Autodesk Inventor part; units mm, degrees
ref_plane "YZ Plane" through (0, 0, 0) normal (1, 0, 0) x (0, 1, 0)
ref_plane "XZ Plane" through (0, 0, 0) normal (0, 1, 0) x (-1, 0, 0)
ref_plane "XY Plane" through (0, 0, 0) normal (0, 0, 1) x (1, 0, 0)
sketch "スケッチ1" plane through (0, 0, 0) normal (0, 0, 1) x (1, 0, 0)
  line L0 (-28, -21) -> (28.6, -21)
  line L1 (28.6, -21) -> (28.6, 21)
  line L2 (28.6, 21) -> (-28, 21)
  line L3 (-28, 21) -> (-28, -21)
  point P0 (0, 0)
  dimension "d1" = 42
  dimension "d28" = 28
  dimension "d29" = 28.6
  dimension "d32" = 21
extrude "プレート1" add sketch "スケッチ1" along normal blind 2
sketch "スケッチ2" plane through (0, 0, 2) normal (0, 0, 1) x (1, 0, 0)
  line L0 (-24, -5) -> (24.6, -5)
  line L1 (24.6, -5) -> (24.6, 5)
  line L2 (24.6, 5) -> (-24, 5)
  line L3 (-24, 5) -> (-24, -5)
  line L4 (-24, -5) -> (24.6, 5) construction
  line L5 (24.6, -5) -> (-24, 5) construction
  line L6 (28.6, -21) -> (-28, -21)
  line L7 (-28, -21) -> (-28, 21)
  line L8 (28.6, -21) -> (-28, -21)
  line L9 (28.6, 21) -> (28.6, -21)
  line L10 (-28, 21) -> (28.6, 21)
  circle A0 centre (-10, 0) radius 7
  point P0 (0.3, 0)
  point P1 (0.3, 0)
  point P2 (0.3, 0)
  point P3 (0, 0)
  dimension "d3" = 48.6
  dimension "d5" = 10
  dimension "d16" = 14
  dimension "d31" = 14
  dimension "d33" = 4
  dimension "d34" = 0
hole "穴1" at (24.6, 5, 2) at (24.6, -5, 2) at (-24, 5, 2) at (-24, -5, 2) direction (0, 0, -1) diameter 4.3 end through all
extrude "押し出し1" cut sketch "スケッチ2" against normal blind 10 contours A0 L2 L0 | L0 A0 | A0 L2
sketch "スケッチ3" plane through (0, 0, 2) normal (0, 0, 1) x (1, 0, 0)
  line L0 (-28, 21) -> (28.6, 21)
  line L1 (-28, -21) -> (-28, 21)
  line L2 (28.6, -21) -> (-28, -21)
  line L3 (28.6, 21) -> (28.6, -21)
  line L4 (24.6, 17) -> (-24, 17)
  line L5 (-24, 17) -> (-24, -17)
  line L6 (-24, -17) -> (24.6, -17)
  line L7 (24.6, -17) -> (24.6, 17)
  point P0 (0, 0)
  dimension "d19" = 4
hole "穴2" at (-24, 17, 2) at (-24, -17, 2) at (24.6, 17, 2) at (24.6, -17, 2) direction (0, 0, -1) diameter 4.3 end through all
fillet "コーナーR1" radius 4 4 edges at (28.6, 21, 1) (-28, 21, 1) (-28, -21, 1) (28.6, -21, 1)
equation "\"d14\" = Thickness"
equation "\"d2\" = Thickness"
equation "\"BendRadius\" = Thickness"
equation "\"BendReliefWidth\" = Thickness"
equation "\"BendReliefDepth\" = 0.5 * Thickness"
equation "\"CornerReliefSize\" = 4 * Thickness"
equation "\"MinimumRemnant\" = 2 * Thickness"
equation "\"TransitionRadius\" = BendRadius"
equation "\"JacobiRadiusSize\" = BendRadius"
equation "\"GapSize\" = Thickness"
properties part number "s_carbon_plate4" material "CFRP"
Could you check a few things on this model? Use its own coordinates, in mm. Coordinates: 2 decimals unless noted, no trailing zeros. Loops run counter-clockwise (first coordinate to the right, second up) from the corner with the lowest first, then second, coordinate; pieces in that order, holes last. Notation, with made-up numbers: M -15.75,67 L 22.25,67 A16 ccw 22.25,95 Z; hole C 58.25,-9.5 d7. An arc over 180 degrees is marked long. Put each result on its own line as item: value. Start each with the question number.
(1) Thinking about a two-plate mould opening in X: for faces 1 (the face through (27.397, -19.859, 1.014)), 2 (the face through (0, 0, 2)), 3 (the face through (-3.534, -2.681, 1.014)), which applies, pulls with the +X half, pulls with the -X half, needs draft (parallel to the pull), parting line crosses it, or undercut?
(2) I need wall thicknesses on line 1 (X direction, y = -17, z = 1.4); line 2 (Y direction, x = -24, z = 1.1); line 3 (X direction, y = -5, z = 0.55). Which ranges of each line are inside material? Lowest first, please. Write a range as from..to.
(3) Suppose I cut it at C-C on y = -5. Please give me the cut outline in (x, z).
(4) Suppose I cut it at B-B on z = 0.8. Count the separate pieces of the cut face and the enclosed holes in it, then the cut area to 3 significant figures.
(5) Suppose I cut it at A-A on x = -10. Please give me the cut outline in (y, z).
Solutions:
1. face 1: pulls with the +X half
1. face 2: needs draft
1. face 3: undercut
2. line 1: x = -28..-26.15, -21.85..22.45, 26.75..28.6
2. line 2: y = -21..-19.15, -14.85..-7.15, -2.85..2.85, 7.15..14.85, 19.15..21
2. line 3: x = -28..-26.15, -21.85..-14.9, -5.1..22.45, 26.75..28.6
3. outline: M -28,0 L -26.15,0 L -26.15,2 L -28,2 Z; M -21.85,0 L -14.9,0 L -14.9,2 L -21.85,2 Z; M -5.1,0 L 22.45,0 L 22.45,2 L -5.1,2 Z; M 26.75,0 L 28.6,0 L 28.6,2 L 26.75,2 Z
4. separate pieces: 1
4. enclosed holes: 9
4. area: 2,090 mm2
5. outline: M -21,0 L -7,0 L -7,2 L -21,2 Z; M 7,0 L 21,0 L 21,2 L 7,2 Z
